```python
from build123d import *

# Parameters (mm, degrees)
EXTRUDE_1_DEPTH     = 30
SKETCH_2_R          = 2
CUT_EXTRUDE_1_DEPTH = 196.491190428


with BuildPart() as part:
    # 草图1 → 凸台-拉伸1 (new body)
    with BuildSketch(Plane.XY):
        with BuildLine():
            Line((150, 25), (-150, 25))
            Line((-150, 25), (-150, -25))
            ThreePointArc((-150, -25), (0, -11.248129774), (150, -25))
            ThreePointArc((150, -25), (133.956439237, 0), (150, 25))
        make_face()
        with BuildLine():
            ThreePointArc((-150, 25), (0, 40.153077165), (150, 25))
            Line((150, 25), (-150, 25))
        make_face()
        with BuildLine():
            ThreePointArc((188.956439237, 0), (176.309013441, 23.14413618), (150, 25))
            Line((150, 25), (150, -25))
            ThreePointArc((150, -25), (176.309013441, -23.14413618), (188.956439237, 0))
        make_face()
        with BuildLine():
            Line((150, -25), (150, 25))
            ThreePointArc((150, 25), (133.956439237, 0), (150, -25))
        make_face()
    extrude(amount=EXTRUDE_1_DEPTH)

    # 草图2 → 切除-拉伸1 (cut, through all)
    with BuildSketch(Plane.XY.offset(30)):
        with Locations((178.706439237, 0)):
            Circle(SKETCH_2_R)
        with Locations((170.081439237, -14.938938215)):
            Circle(SKETCH_2_R)
        with Locations((152.831439237, -14.938938215)):
            Circle(SKETCH_2_R)
        with Locations((144.206439237, 0)):
            Circle(SKETCH_2_R)
        with Locations((152.831439237, 14.938938215)):
            Circle(SKETCH_2_R)
        with Locations((170.081439237, 14.938938215)):
            Circle(SKETCH_2_R)
    extrude(amount=-CUT_EXTRUDE_1_DEPTH, mode=Mode.SUBTRACT)


solid = part.part
```
Geometry check sheet. Reference: the model listing, model coordinates, mm. Give positions to 0.01 mm unless a question says otherwise; leave off trailing zeros. Order: outer loops, then holes, each group sorted by start corner. A loop starts at its lowest first (then second) coordinate and runs counter-clockwise, first axis right, second up. Notation, with made-up numbers: (50, -22) - (92, -22) arc R22 ccw to (92, 17) - close; hole circle Ø3 at (52, -40). An arc over 180 degrees is marked (long way). Write item = value, one per line. Start each with the question number.
1) Scan lines: L1, parallel to X at y = 16, z = 9.5; L2, parallel to Y at x = -5.5, z = 3.25; L3, parallel to Y at x = -96.5, z = 22.75. Record each from-to range of solid material in increasing order.
2) Section check C-C (x = 56.5). Enter the section's corners in (y, z), then the cut area to 3 significant figures.
3) Section check B-B (x = -58). Enter the section's corners in (y, z).
4) Gauge pin test, flat ends, axial feed: pin 1 Ø8 at (x, y) = (-52.5, -10.5) entering from -Z; pin 2 Ø3 at (x, y) = (170.08, 14.94) entering from +Z; pin 3 Ø1.5 at (y, z) = (-9, 15.5) entering from +X. Record the tip position at first contact, or that the pin passes through.
5) Section check A-A (z = 25). Enter the section's corners in (x, y), then the cut area to 3 significant figures.
6) Draft check along X on faces 1 (the flat face through (17, 7, 30)), 2 (the cylindrical face through (-2.11, -11.25, 14.79)), 3 (the flat face through (-150, 0, 15)). Enter one of: released by +X, released by -X, zero draft, split by the parting line, or undercut.
Geometry check:
q1.L1 = -150 to 151.14, 154.53 to 168.39, 171.78 to 183.82
q1.L2 = -11.27 to 40.13
q1.L3 = -16.91 to 33.92
q2.outline = (-13.19, 0) - (38.02, 0) - (38.02, 30) - (-13.19, 30) - close
q2.area = 1,540 mm2
q3.outline = (-13.29, 0) - (37.91, 0) - (37.91, 30) - (-13.29, 30) - close
q4.pin_1 = 0
q4.pin_2 = through
q4.pin_3 = 187.69
q5.outline = (-150, -25) arc R824.95 cw to (150, -25) arc R27.5 ccw (long way) to (150, 25) arc R750 ccw to (-150, 25) - close; hole circle Ø4 at (144.21, 0); hole circle Ø4 at (152.83, -14.94); hole circle Ø4 at (152.83, 14.94); hole circle Ø4 at (170.08, -14.94); hole circle Ø4 at (170.08, 14.94); hole circle Ø4 at (178.71, 0)
q5.area = 17,000 mm2
q6.face_1 = zero draft
q6.face_2 = undercut
q6.face_3 = released by -X
